```python
from build123d import *

# Parameters (mm, degrees)
F0_R     = 4
F0_R_2   = 3
F1_DEPTH = 2
F2_START = 1
F0_R_3   = 2
F2_DEPTH = 5
F3_START = 5
F0_R_4   = 1
F3_DEPTH = 25
F5_D     = 2
F5_DEPTH = 4.001
F6_D     = 2


with BuildPart() as f1:
    # F0 (on Front) → F1 (new body)
    with BuildSketch(Plane.XZ):
        Circle(F0_R)
        Circle(F0_R_2, mode=Mode.SUBTRACT)
    extrude(amount=F1_DEPTH)

    # F0 (on Front) → F2 (join)
    with BuildSketch(Plane.XZ.offset(F2_START)):
        Circle(F0_R_2)
        Circle(F0_R_3, mode=Mode.SUBTRACT)
    extrude(amount=F2_DEPTH)

    # F0 (on Front) → F3 (join)
    with BuildSketch(Plane.XZ.offset(F3_START)):
        Circle(F0_R_3)
        Circle(F0_R_4, mode=Mode.SUBTRACT)
    extrude(amount=F3_DEPTH)

    # F5 (through all, one way)
    with BuildSketch(Plane.XY):
        with Locations((0, -28.5)):
            Circle(F5_D / 2)
    extrude(amount=-F5_DEPTH, mode=Mode.SUBTRACT)

    # F6 (through all)
    with Locations(Plane(origin=(0, 0, 0), x_dir=(1, 0, 0), z_dir=(0, 0, -1))):
        with Locations((0, 28.5)):
            Hole(F6_D / 2)


solid = f1.part
```
Geometry: final body of the model. Coordinates: model frame, mm. A direction names the side the tool comes from. Coordinates: 2 decimals unless noted, no trailing zeros. Write each loop counter-clockwise with the first axis right and the second up, starting at its lowest first coordinate (ties: lowest second). Pieces come first, ordered by that corner, then holes. Notation, with made-up numbers: M 24.25,37.5 L 46.25,37.5 A13 cw 46.25,48.5 Z; hole C -2,15.5 d4. An arc over 180 degrees is marked long. Answer as CSV lines item,"result". Start each with the question number.
Q1. Mould query, pull axis Z, two halves, no side actions, for faces 4 (the flat face through (1, -1, -2)), 5 (the cylindrical face through (-3, -4, 0)), 6 (the flat face through (1, -6, -2)). Classes: released by +Z, released by -Z, zero draft, split by the parting line, or undercut.
Q2. Cut plane C-C on y = -21. Return the cut outline in (x, z).
Q3. Reachability of faces 1 (the cylindrical face through (0, -18, 2)), 2 (the cylindrical face through (-0.217, -29.476, -1.208)), 3 (the cylindrical face through (0, -3, -2)) from +Z, -Z, +X, -X, +Y, -Y: full face, straight path, thin tool, end or side. Return the list, or none.
Q4. Cut plane D-D on x = 1.5. Return the cut outline in (y, z), then the cut area to 3 significant figures.
Q5. Cut plane A-A on x = 0. Count the separate pieces of the cut face and the enclosed holes in it, then the cut area to 3 significant figures.
Q6. Cut plane B-B on z = -0.5. Return the cut outline in (x, y), then the cut area to 3 significant figures.
Q7. Line query: line 1 (Y direction, x = 3.5, z = 1.5); line 2 (Z direction, x = 0, y = -26.5); line 3 (Y direction, x = -1, z = 2.5). Output: solid intervals per line, ascending. Write a range as from..to.
Q8. Pin query (flat end, axial travel): P1, Ø1.2, axis at x = 0, z = -1, coming from the +Y side; P2, Ø3, axis at x = 0.5, y = -8.5, coming from the +Z side; P3, Ø1.5, axis at y = -25, z = 0.5, coming from the +X side; P4, Ø1.6, axis at x = 0, y = -28.5, coming from the +Z side. Return the tip coordinate at first contact, or that it passes through.
Findings below:
1,face 4,"undercut"
1,face 5,"split by the parting line"
1,face 6,"zero draft"
2,outline,"C 0,0 d4; hole C 0,0 d2"
3,face 1,"-Y"
3,face 2,"+Z, -Z"
3,face 3,"+Y"
4,outline,"M -30,-1.32 L -6,-1.32 L -6,-2.6 L -2,-2.6 L -2,-3.71 L 0,-3.71 L 0,-2.6 L -1,-2.6 L -1,-1.32 L -5,-1.32 L -5,1.32 L -1,1.32 L -1,2.6 L 0,2.6 L 0,3.71 L -2,3.71 L -2,2.6 L -6,2.6 L -6,1.32 L -30,1.32 Z"
4,area,"83.3 mm2"
5,separate pieces,"4"
5,enclosed holes,"0"
5,area,"60.0 mm2"
6,outline,"M -3.97,-2 L -2.96,-2 L -2.96,-6 L -1.94,-6 L -1.94,-30 L -0.87,-30 L -0.87,-29 A1 cw -0.87,-28 L -0.87,-5 L -1.94,-5 L -1.94,-1 L -2.96,-1 L -2.96,0 L -3.97,0 Z; M 0.87,-30 L 1.94,-30 L 1.94,-6 L 2.96,-6 L 2.96,-2 L 3.97,-2 L 3.97,0 L 2.96,0 L 2.96,-1 L 1.94,-1 L 1.94,-5 L 0.87,-5 L 0.87,-28 A1 cw 0.87,-29 Z"
6,area,"67.6 mm2"
7,line 1,"y = -2..0"
7,line 2,"z = -2..-1, 1..2"
7,line 3,"y = -6..-1"
8,P1,"stops at y = -5"
8,P2,"stops at z = 2"
8,P3,"stops at x = 2"
8,P4,"passes through"
